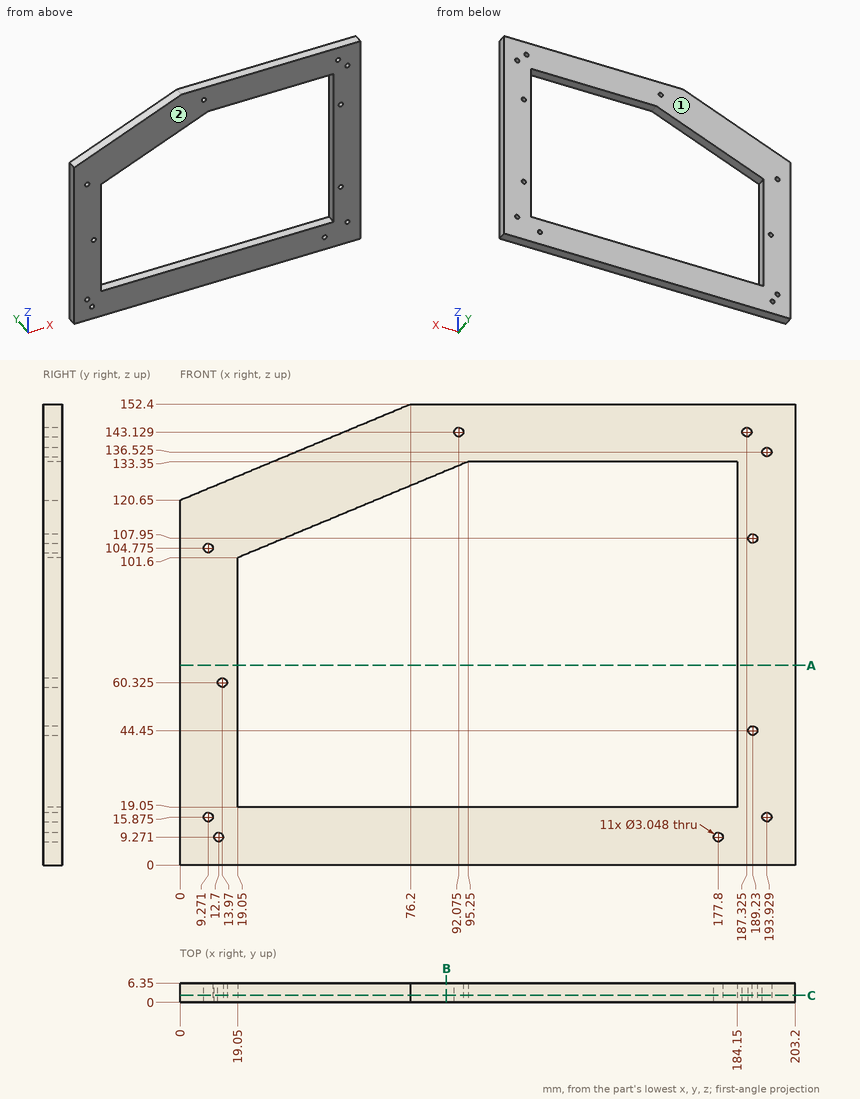
Input: dimensioned drawing with shaded views. Units: mm. Origin: part minimum x, y, z. Round coordinates to 2 decimals unless told otherwise and drop trailing zeros. Order: outer loops, then holes, each group sorted by start corner. A loop starts at its lowest first (then second) coordinate and runs counter-clockwise, first axis right, second up. Notation, with made-up numbers: (84, 47) - (107, 47) arc R17 ccw to (107, 67) - close; hole circle Ø7 at (-23.5, 36.5). An arc over 180 degrees is marked (long way). Use CSV: the item, a comma, the result in double quotes. Start each with the question number.
Q1. Section query C-C (y = 2.25). State how many separate pieces and enclosed holes the cut face has, and give its area (3 significant figures).
Q2. First-contact query: pin 1 (2 mm diameter, centred on x = 72.5, y = 2.5, fed in from +Z) (3 decimals). Flat tip, straight axial feed; report the tip coordinate or a pass-through.
Q3. Mould query, pull axis Y, two halves, no side actions, for the marked faces 1 and 2. Classes: +Y half, -Y half, draft (parallel to the pull), parting line (faces both ways), or undercut.
Q4. Section query B-B (x = 88). Return loops of the section in (y, z), and give its area (3 significant figures).
Q5. Section query A-A (z = 66). Return loops of the section in (x, y), and give its area (3 significant figures).
Q6. Material intervals for line 1 along X through (y, z) = (1.5, 44.45); line 2 along Z through (x, y) = (181, 3); line 3 along X through (y, z) = (4.5, 94.5), sorted ascending. Write a range as from..to.
Result set:
1,separate pieces,"1"
1,enclosed holes,"12"
1,area,"12,000 mm2"
2,pin 1,"stops at z = 151.275"
3,face 1,"+Y half"
3,face 2,"-Y half"
4,outline,"(0, 0) - (6.35, 0) - (6.35, 19.05) - (0, 19.05) - close; (0, 130.33) - (6.35, 130.33) - (6.35, 152.4) - (0, 152.4) - close"
4,area,"261 mm2"
5,outline,"(0, 0) - (19.05, 0) - (19.05, 6.35) - (0, 6.35) - close; (184.15, 0) - (203.2, 0) - (203.2, 6.35) - (184.15, 6.35) - close"
5,area,"242 mm2"
6,line 1,"x = 0..19.05, 184.15..187.71, 190.75..203.2"
6,line 2,"z = 0..19.05, 133.35..152.4"
6,line 3,"x = 0..19.05, 184.15..203.2"
